Work out the finished part from the listing and answer in its coordinate system (mm). A direction names the side the tool comes from. Coordinates: 2 decimals unless noted, no trailing zeros. Write each loop counter-clockwise with the first axis right and the second up, starting at its lowest first coordinate (ties: lowest second). Pieces come first, ordered by that corner, then holes. Notation, with made-up numbers: (-10, 22) - (16, 22) arc R26 cw to (16, 51) - close; hole circle Ø6 at (2, 48.25). An arc over 180 degrees is marked (long way). Use one line per item in the form item = value. Start each with the question number.
Item 1: Determine the mould class of faces 1 (the flat face through (12, -2, 0)), 2 (the cylindrical face through (26, 0, 0)), 3 (the cylindrical face through (21, 0, 0)) for opening direction Y: released by +Y, released by -Y, zero draft, split by the parting line, or undercut.
Item 2: Given pin 1 (2 mm diameter, centred on x = 9.5, z = -0.5, fed in from -Y); pin 2 (0.5 mm diameter, centred on y = -2.5, z = 0.5, fed in from -X); pin 3 (0.8 mm diameter, centred on y = -2.5, z = 0, fed in from +X), each flat-ended and moving along its own axis, determine where each tip first touches the part or whether it passes through.
Item 3: For faces 4 (the flat face through (4, -2.5, 0)), 5 (the flat face through (12, 0, 2)), 6 (the flat face through (11, 2, 0)), determine the directions among +Z, -Z, +X, -X, +Y, -Y from which every point of the face is accessible in a straight line to the end or side of a thin tool.
Item 4: A cutting plane is placed at D-D (x = 8.5). Write down the section's boundary in (y, z), then the cut area to 3 significant figures.
Item 5: A cutting plane is placed at B-B (z = 1.65). Write down the section's boundary in (x, y).
Item 6: Consider probe 1 along Y at (x, z) = (0, 0.55); probe 2 along X at (y, z) = (0.35, 0.4); probe 3 along X at (y, z) = (-0.75, -0.8). Determine where each line is inside the solid, lowest interval first.
Item 7: A cutting plane is placed at A-A (y = 0). Write down the section's boundary in (x, z).
Item 8: A cutting plane is placed at C-C (y = 2.6). Write down the section's boundary in (x, z), then the cut area to 3 significant figures.
from build123d import *

# Parameters (mm, degrees)
SKETCH_1_R      = 2
EXTRUDE_1_DEPTH = 2


with BuildPart() as part:
    # 草图1 → 凸台-拉伸1 (new, symmetric)
    with BuildSketch(Plane.XY):
        with BuildLine():
            Line((0, 3), (4, 3))
            Line((4, 3), (4, 2))
            Line((4, 2), (19, 2))
            Line((19, 2), (19, 3))
            Line((19, 3), (23, 3))
            ThreePointArc((23, 3), (26, 0), (23, -3))
            Line((23, -3), (19, -3))
            Line((19, -3), (19, -2))
            Line((19, -2), (4, -2))
            Line((4, -2), (4, -3))
            Line((4, -3), (0, -3))
            ThreePointArc((0, -3), (-3, 0), (0, 3))
        make_face()
        Circle(SKETCH_1_R, mode=Mode.SUBTRACT)
        with Locations((23, 0)):
            Circle(SKETCH_1_R, mode=Mode.SUBTRACT)
    extrude(amount=EXTRUDE_1_DEPTH, both=True)


solid = part.part
Answer:
q1.face_1 = released by -Y
q1.face_2 = split by the parting line
q1.face_3 = undercut
q2.pin_1 = -2
q2.pin_2 = -1.98
q2.pin_3 = 25.14
q3.face_4 = +Z, -Z, -Y
q3.face_5 = +Z, +X, -X, +Y, -Y
q3.face_6 = +Z, -Z, +Y
q4.outline = (-2, -2) - (2, -2) - (2, 2) - (-2, 2) - close
q4.area = 16.0 mm²
q5.outline = (0, -3) - (4, -3) - (4, -2) - (19, -2) - (19, -3) - (23, -3) arc R3 ccw to (23, 3) - (19, 3) - (19, 2) - (4, 2) - (4, 3) - (0, 3) arc R3 ccw to start; hole circle Ø4 at (0, 0); hole circle Ø4 at (23, 0)
q6.probe_1 = -3 to -2, 2 to 3
q6.probe_2 = -2.98 to -1.97, 1.97 to 21.03, 24.97 to 25.98
q6.probe_3 = -2.9 to -1.85, 1.85 to 21.15, 24.85 to 25.9
q7.outline = (-3, -2) - (-2, -2) - (-2, 2) - (-3, 2) - close; (2, -2) - (21, -2) - (21, 2) - (2, 2) - close; (25, -2) - (26, -2) - (26, 2) - (25, 2) - close
q8.outline = (-1.5, -2) - (4, -2) - (4, 2) - (-1.5, 2) - close; (19, -2) - (24.5, -2) - (24.5, 2) - (19, 2) - close
q8.area = 44.0 mm²
